Source: three-view drawing plus pictorial views. Frame: mm from the lowest corner of the part. Give positions to 0.01 mm unless a question says otherwise; leave off trailing zeros. Order: outer loops, then holes, each group sorted by start corner. A loop starts at its lowest first (then second) coordinate and runs counter-clockwise, first axis right, second up.
1) Section A-A, the plane x = 41. Return loops of the section in (y, z).
2) Section D-D, the plane y = 1. Give the number of separate pieces and of enclosed holes in the cut face, plus the area to 3 significant figures.
3) Section C-C, the plane z = 6. Return loops of the section in (x, y) (1 decimal), plus the area to 3 significant figures.
4) Section B-B, the plane x = 30. Return loops of the section in (y, z), plus the area to 3 significant figures.
5) Material intervals for line 1 (Z direction, x = 50, y = 0.85) (1 decimal); line 2 (Z direction, x = 50, y = 2.7) (1 decimal); line 3 (X direction, y = 4.75, z = 21) (1 decimal), sorted ascending.
6) First-contact query: P1, Ø3, axis at x = 48, z = 4.5, coming from the -Y side; P2, Ø2, axis at x = 30, z = 21.57, coming from the -Y side. Flat tips, straight axial feed; report the tip coordinate or a pass-through.
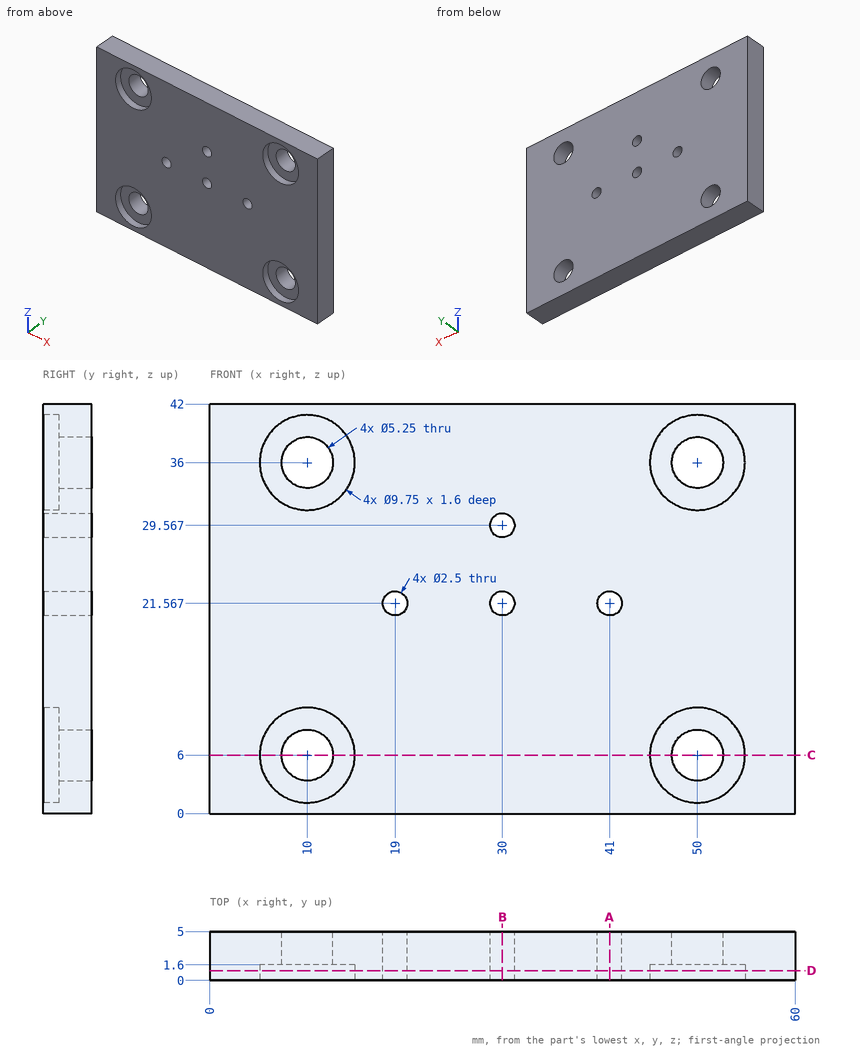
From the geometry:
1. outline: (0, 0) - (5, 0) - (5, 20.32) - (0, 20.32) - close; (0, 22.82) - (5, 22.82) - (5, 42) - (0, 42) - close
2. separate pieces: 1
2. enclosed holes: 8
2. area: 2,200 mm2
3. outline: (0, 0) - (5.1, 0) - (5.1, 1.6) - (7.4, 1.6) - (7.4, 5) - (0, 5) - close; (12.6, 1.6) - (14.9, 1.6) - (14.9, 0) - (45.1, 0) - (45.1, 1.6) - (47.4, 1.6) - (47.4, 5) - (12.6, 5) - close; (52.6, 1.6) - (54.9, 1.6) - (54.9, 0) - (60, 0) - (60, 5) - (52.6, 5) - close
3. area: 233 mm2
4. outline: (0, 0) - (5, 0) - (5, 20.32) - (0, 20.32) - close; (0, 22.82) - (5, 22.82) - (5, 28.32) - (0, 28.32) - close; (0, 30.82) - (5, 30.82) - (5, 42) - (0, 42) - close
4. area: 185 mm2
5. line 1: z = 0 to 1.1, 10.9 to 31.1, 40.9 to 42
5. line 2: z = 0 to 3.4, 8.6 to 33.4, 38.6 to 42
5. line 3: x = 0 to 17.9, 20.1 to 28.9, 31.1 to 39.9, 42.1 to 60
6. P1: stops at y = 1.6
6. P2: passes through
